Autodesk Inventor part; units mm, degrees
ref_plane "magnet_to_mgplate_XY" through (-3, 8, 0) normal (1, 0, 0) x (0, 0, -1)
ref_plane "magnet_to_mgplate_YZ" through (-3, 8, 0) normal (0, 0, -1) x (0, 1, 0)
ref_plane "magnet_to_mgplate_ZX" through (-3, 8, 0) normal (0, 1, 0) x (1, 0, 0)
sketch "Sketch_2" plane through (0, 0, 0) normal (0, 1, 0) x (-1, 0, 0)
  line L0 (0, -26.25) -> (0, 26.25)
  arc A0 (0, 26.25) -> (-2, 28.25) centre (-2, 26.25) ccw
  line L1 (-2, 28.25) -> (-21.5, 28.25)
  arc A1 (-21.5, 28.25) -> (-23.5, 26.25) centre (-21.5, 26.25) ccw
  line L2 (-23.5, 26.25) -> (-23.5, -26.25)
  arc A2 (-23.5, -26.25) -> (-21.5, -28.25) centre (-21.5, -26.25) ccw
  line L3 (-21.5, -28.25) -> (-2, -28.25)
  arc A3 (-2, -28.25) -> (0, -26.25) centre (-2, -26.25) ccw
  arc A4 (-9.5, 20.75) -> (-9.5, 24.25) centre (-9.5, 22.5) ccw
  line L4 (-9.5, 24.25) -> (-14, 24.25)
  arc A5 (-14, 24.25) -> (-14, 20.75) centre (-14, 22.5) ccw
  line L5 (-14, 20.75) -> (-9.5, 20.75)
  arc A6 (-9.5, -24.25) -> (-9.5, -20.75) centre (-9.5, -22.5) ccw
  line L6 (-9.5, -20.75) -> (-14, -20.75)
  arc A7 (-14, -20.75) -> (-14, -24.25) centre (-14, -22.5) ccw
  line L7 (-14, -24.25) -> (-9.5, -24.25)
extrude "Extrusion1" add sketch "Sketch_2" along normal blind 15.5
sketch "Sketch_1" plane through (0, 0, 0) normal (1, 0, 0) x (0, 1, 0)
  line L0 (-10, 50) -> (-10, -50)
  line L1 (-10, -50) -> (30, -50)
  line L2 (30, -50) -> (30, 50)
  line L3 (30, 50) -> (-10, 50)
  line L4 (0, 28.25) -> (0, -28.25)
  arc A0 (0, -28.25) -> (2, -26.25) centre (0, -26.25) ccw
  line L5 (2, -26.25) -> (2, -18.75)
  arc A1 (4, -16.75) -> (2, -18.75) centre (4, -18.75) ccw
  line L6 (4, -16.75) -> (13.5, -16.75)
  arc A2 (13.5, -16.75) -> (15.5, -14.75) centre (13.5, -14.75) ccw
  line L7 (15.5, -14.75) -> (15.5, 14.75)
  arc A3 (15.5, 14.75) -> (13.5, 16.75) centre (13.5, 14.75) ccw
  line L8 (13.5, 16.75) -> (4, 16.75)
  arc A4 (2, 18.75) -> (4, 16.75) centre (4, 18.75) ccw
  line L9 (2, 18.75) -> (2, 26.25)
  arc A5 (2, 26.25) -> (0, 28.25) centre (0, 26.25) ccw
extrude "Extrusion2" cut sketch "Sketch_1" along normal blind 24
sketch "Sketch_3" plane through (0, 0, 0) normal (1, 0, 0) x (0, 1, 0)
  line L0 (3, 10.75) -> (3, -10.75)
  line L1 (3, -10.75) -> (5, -10.75)
  line L2 (5, -10.75) -> (5, 10.75)
  line L3 (5, 10.75) -> (3, 10.75)
extrude "Extrusion3" add sketch "Sketch_3" against normal blind 3
sketch "Sketch_4" plane through (0, 0, 0) normal (1, 0, 0) x (0, 1, 0)
  line L0 (11.5, 10.75) -> (11.5, -10.75)
  line L1 (11.5, -10.75) -> (13.5, -10.75)
  line L2 (13.5, -10.75) -> (13.5, 10.75)
  line L3 (13.5, 10.75) -> (11.5, 10.75)
extrude "Extrusion4" add sketch "Sketch_4" against normal blind 3
ref_plane "magnet_to_mgplate_XY" through (-3, 8, 0) normal (1, 0, 0) x (0, 0, -1)
ref_plane "magnet_to_mgplate_YZ" through (-3, 8, 0) normal (0, 0, -1) x (0, 1, 0)
ref_plane "magnet_to_mgplate_ZX" through (-3, 8, 0) normal (0, 1, 0) x (1, 0, 0)
ref_plane "to_plate_XY" through (11.9, 0, -22.5) normal (0, 1, 0) x (1, 0, 0)
ref_plane "to_plate_YZ" through (11.9, 0, -22.5) normal (1, 0, 0) x (0, 0, -1)
ref_plane "to_plate_ZX" through (11.9, 0, -22.5) normal (0, 0, -1) x (0, 1, 0)
properties part number "MGCE15-5"
Here's how the part is built. I have some questions about the finished solid (model axes, mm). A direction names the side the tool comes from. Round coordinates to 2 decimals unless told otherwise and drop trailing zeros. Loops run counter-clockwise (first coordinate to the right, second up) from the corner with the lowest first, then second, coordinate; pieces in that order, holes last. Notation, with made-up numbers: (49.5, 3) -> (59.5, 3) arc R14 ccw to (59.5, 16) -> close; hole circle Ø7 at (10.5, 76.25). An arc over 180 degrees is marked (long way). Answer as CSV lines item,"result".
1. If we section it at A-A on x = 12.5: Please give me the cut outline in (y, z).
Final values:
outline,"(0, -28.25) arc R2 ccw to (2, -26.25) -> (2, -24.25) -> (0, -24.25) -> close; (0, -20.75) -> (2, -20.75) -> (2, -18.75) arc R2 cw to (4, -16.75) -> (13.5, -16.75) arc R2 ccw to (15.5, -14.75) -> (15.5, 14.75) arc R2 ccw to (13.5, 16.75) -> (4, 16.75) arc R2 cw to (2, 18.75) -> (2, 20.75) -> (0, 20.75) -> close; (0, 24.25) -> (2, 24.25) -> (2, 26.25) arc R2 ccw to (0, 28.25) -> close"
2. If I drill on L1, parallel to X at y = 10.25, z = -2; L2, parallel to Y at x = 1, z = 22.5; L3, parallel to Z at x = 21.5, y = 6, over which ranges is the centre line in solid material (lowest first)?
Final values:
L1,"x = 0 to 23.5"
L2,"y = 0 to 2"
L3,"z = -16.75 to 16.75"
3. For pin 1 (7.5 mm diameter, centred on x = 14.5, y = 7, fed in from -Z); pin 2 (3 mm diameter, centred on y = 3, z = 19, fed in from +X); pin 3 (4 mm diameter, centred on x = 11, y = 5, fed in from -Z); pin 4 (1 mm diameter, centred on x = -2, y = 4, fed in from +Z), each with a flat end and sliding along its axis, tell me the tip position at first contact or that it passes through.
Final values:
pin 1,"stops at z = -16.9"
pin 2,"stops at x = 23.5"
pin 3,"stops at z = -17.02"
pin 4,"stops at z = 10.75"
4. If we section it at D-D on z = 3.5: Please give me the cut outline in (x, y), plus the area to 3 significant figures.
Final values:
outline,"(-3, 3) -> (0, 3) -> (0, 0) -> (23.5, 0) -> (23.5, 15.5) -> (0, 15.5) -> (0, 13.5) -> (-3, 13.5) -> (-3, 11.5) -> (0, 11.5) -> (0, 5) -> (-3, 5) -> close"
area,"376 mm^2"
5. If we section it at C-C on x = 4.5: Please give me the cut outline in (y, z), plus the area to 3 significant figures.
Final values:
outline,"(0, -28.25) arc R2 ccw to (2, -26.25) -> (2, -18.75) arc R2 cw to (4, -16.75) -> (13.5, -16.75) arc R2 ccw to (15.5, -14.75) -> (15.5, 14.75) arc R2 ccw to (13.5, 16.75) -> (4, 16.75) arc R2 cw to (2, 18.75) -> (2, 26.25) arc R2 ccw to (0, 28.25) -> close"
area,"564 mm^2"
6. Which directions (+Z, -Z, +X, -X, +Y, -Y) give clear straight access to the entire face, cutting with the end or side of a thin tool? Please do faces 1 (the face through (12, 9, -16.75)), 2 (the face through (-1, 4, 10.75)), 3 (the face through (12, 1, -24.25)), 4 (the face through (12, 9, 16.75)), 5 (the face through (-1, 12, -10.75)).
Final values:
face 1,"-Z, +X, -X, +Y"
face 2,"+Z, -X, +Y, -Y"
face 3,"+Y, -Y"
face 4,"+Z, +X, -X, +Y"
face 5,"-Z, -X, +Y, -Y"
7. If we section it at B-B on z = -22.5: Please give me the cut outline in (x, y).
Final values:
outline,"(0, 0) -> (7.75, 0) -> (7.75, 2) -> (0, 2) -> close; (15.75, 0) -> (23.5, 0) -> (23.5, 2) -> (15.75, 2) -> close"
8. Thinking about a two-plate mould opening in Y: for faces 6 (the face through (11.59, 14.93, -16.15)), 7 (the face through (-1, 11.5, 0)), 8 (the face through (15.75, 0.99, 22.46)), 9 (the face through (-1, 3, 0)), which applies, released by +Y, released by -Y, zero draft, split by the parting line, or undercut?
Final values:
face 6,"released by +Y"
face 7,"undercut"
face 8,"zero draft"
face 9,"released by -Y"
